Check sheet for the modelled part. Datum: model origin and axes. Units: mm. Round coordinates to 2 decimals unless told otherwise and drop trailing zeros. Write each loop counter-clockwise with the first axis right and the second up, starting at its lowest first coordinate (ties: lowest second). Pieces come first, ordered by that corner, then holes. Notation, with made-up numbers: M 42,55.5 L 76,55.5 A25 ccw 76,80.5 Z; hole C 54,53 d10. An arc over 180 degrees is marked long. One line per item, written item: value.
Autodesk Inventor part; units mm, degrees
ref_plane "YZ Plane" through (0, 0, 0) normal (1, 0, 0) x (0, 1, 0)
ref_plane "XZ Plane" through (0, 0, 0) normal (0, 1, 0) x (-1, 0, 0)
ref_plane "XY Plane" through (0, 0, 0) normal (0, 0, 1) x (1, 0, 0)
sketch "Sketch_1" plane through (0, 0, 0) normal (0, 0, 1) x (1, 0, 0)
  line L0 (16, 0) -> (0, 0)
  line L1 (0, 0) -> (0, 5.6)
  arc A0 (0.4, 6) -> (0, 5.6) centre (0.4, 5.6) ccw
  line L2 (0.4, 6) -> (7.2859, 6)
  arc A1 (7.2859, 6) -> (8.7141, 6) centre (8, 6.7) ccw
  line L3 (8.7141, 6) -> (15.6, 6)
  arc A2 (16, 5.6) -> (15.6, 6) centre (15.6, 5.6) ccw
  line L4 (16, 5.6) -> (16, 0)
  line L5 (16, 0) -> (0, 0)
revolve "Revolution1" add sketch "Sketch_1" angle 360 about axis through (16, 0, 0) along (1, 0, 0)
sketch "Sketch2" plane through (16, 0, 0) normal (1, 0, 0) x (0, 0, -1)
  point P0 (0, 0)
hole "Hole1" at (16, 0, 0) direction (-1, 0, 0) diameter 6 depth 16
properties part number "LMUT6" material "鉄、鋳鉄"
Q1. Sectioned sample at C-C on x = 14.75. Enter the section's corners in (y, z), and give its area (3 significant figures).
Completed:
outline: C 0,0 d12; hole C 0,0 d6
area: 84.8 mm^2
Q2. Scan lines: line 1 (Z direction, x = 12, y = 0); line 2 (Z direction, x = 5, y = -2.5); line 3 (Y direction, x = 2, z = -2). Record each from-to range of solid material in increasing order. Write a range as [from, to].
Completed:
line 1: [-6, -3], [3, 6]
line 2: [-5.45, -1.66], [1.66, 5.45]
line 3: [-5.66, -2.24], [2.24, 5.66]
Q3. Sectioned sample at A-A on y = 0. Enter the section's corners in (x, z), and give its area (3 significant figures).
Completed:
outline: M 0,-5.6 A0.4 ccw 0.4,-6 L 7.29,-6 A1 cw 8.71,-6 L 15.6,-6 A0.4 ccw 16,-5.6 L 16,-3 L 0,-3 Z; M 0,3 L 16,3 L 16,5.6 A0.4 ccw 15.6,6 L 8.71,6 A1 cw 7.29,6 L 0.4,6 A0.4 ccw 0,5.6 Z
area: 95.3 mm^2
Q4. Depth check by flat-ended pin: P1, Ø3, axis at x = 11.5, y = -4, coming from the -Z side. Enter the tip coordinate at first touch or a pass-through.
Completed:
P1: z = -5.45
